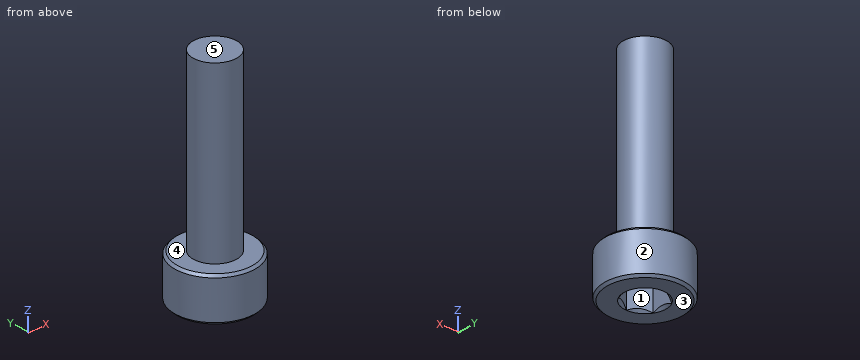
```python
from build123d import *

# Parameters (mm, degrees)
SKETCH1_R          = 1.5
EXTRUDE1_DEPTH     = 12
SKETCH6_R          = 2.75
EXTRUDE2_DEPTH     = 3
CUT_EXTRUDE1_DEPTH = 1.875
CHAMFER1_SIZE      = 0.165


with BuildPart() as part:
    # Sketch1 → Extrude1 (new body)
    with BuildSketch(Plane.XY):
        Circle(SKETCH1_R)
    extrude(amount=-EXTRUDE1_DEPTH)

    # Sketch6 → Extrude2 (add)
    with BuildSketch(Plane(origin=(0, 0, -12), x_dir=(-1, 0, 0), z_dir=(0, 0, -1))):
        Circle(SKETCH6_R)
    extrude(amount=EXTRUDE2_DEPTH)

    # Sketch7 → Cut-Extrude1 (cut)
    with BuildSketch(Plane(origin=(0, 0, -15), x_dir=(-1, 0, 0), z_dir=(0, 0, -1))):
        Polygon((0, 1.443375673), (-1.25, 0.721687836), (-1.25, -0.721687836), (0, -1.443375673), (1.25, -0.721687836), (1.25, 0.721687836), align=None)
    extrude(amount=-CUT_EXTRUDE1_DEPTH, mode=Mode.SUBTRACT)

    # Cut-Extrude2 cone 1 section (through the dimple's axis) → Cut-Extrude2 (revolve, cut)
    with BuildSketch(Plane(origin=(0, 0, -15), x_dir=(0, 1, 0), z_dir=(1, 0, 0))):
        Polygon((0, 0), (1.443375673, 0), (0, 1.443375673), align=None)
    revolve(axis=Axis((0, 0, -15), (0, 0, 1)), mode=Mode.SUBTRACT)

    # Chamfer1
    chamfer1_edges = [part.edges().sort_by_distance(p)[0] for p in [
        (2.75, 0, -12),
        (2.75, 0, -15),
    ]]
    chamfer(chamfer1_edges, length=CHAMFER1_SIZE)

    # Sketch10 → Revolve1 (revolve)
    with BuildSketch(Plane(origin=(0, 0, 0), x_dir=(0, 0, -1), z_dir=(1, 0, 0))):
        Polygon((12, 1.5), (12, 0), (11.253679656, 0), (11.875, 1.5), align=None)
    revolve(axis=Axis((0, 0, -12), (0, 0, 1)))


solid = part.part
```
Work out the finished part from the listing and answer in its coordinate system (mm). Face numbers are marked on the shaded views. A direction names the side the tool comes from. Give positions to 0.01 mm unless a question says otherwise; leave off trailing zeros. Write each loop counter-clockwise with the first axis right and the second up, starting at its lowest first coordinate (ties: lowest second). Pieces come first, ordered by that corner, then holes.
(1) Which of the six approach directions +Z, -Z, +X, -X, +Y, -Y give full straight-line access (tool end or side, diameter ignored) to the marked faces 4 and 5?
Final values:
face 4: +Z
face 5: +Z, +X, -X, +Y, -Y
(2) The mould has two halves that part along Y. Classify the marked faces 1, 2 and 3: pulls with the +Y half, pulls with the -Y half, needs draft (parallel to the pull), parting line crosses it, or undercut.
Final values:
face 1: undercut
face 2: parting line crosses it
face 3: needs draft
(3) The part is cut by section B-B on z = -4.75. Write down the section's boundary in (x, y).
Final values:
outline: circle Ø3 at (0, 0)
(4) Straight lines are drawn through the part: line 1 (Z direction, x = 0.9, y = -1.4); line 2 (Z direction, x = 1.15, y = 0.45) (3 decimals); line 3 (Y direction, x = 0, z = -8.75). For each, find the intervals that lie inside material, in ascending order.
Final values:
line 1: z = -15 to -12
line 2: z = -13.125 to 0
line 3: y = -1.5 to 1.5
(5) Flat-ended cylindrical pins translate along their axes: pin 1 Ø1 at (y, z) = (-1, -2.5) entering from -X; pin 2 Ø1.2 at (x, y) = (-0.5, -0.5) entering from -Z; pin 3 Ø2 at (y, z) = (2, -5.5) entering from +X. Find the tip coordinate at first contact, or state that the pin passes through.
Final values:
pin 1: stops at x = -1.41
pin 2: stops at z = -14.86
pin 3: stops at x = 1.12
(6) The part is cut by section A-A on y = 0. Write down the section's boundary in (x, z) (3 decimals), plus the area to 3 significant figures.
Final values:
outline: (-2.75, -14.835) - (-2.585, -15) - (-1.443, -15) - (-1.25, -14.807) - (-1.25, -13.125) - (1.25, -13.125) - (1.25, -14.807) - (1.443, -15) - (2.585, -15) - (2.75, -14.835) - (2.75, -12.165) - (2.585, -12) - (1.5, -12) - (1.5, 0) - (-1.5, 0) - (-1.5, -12) - (-2.585, -12) - (-2.75, -12.165) - close
area: 47.7 mm2
